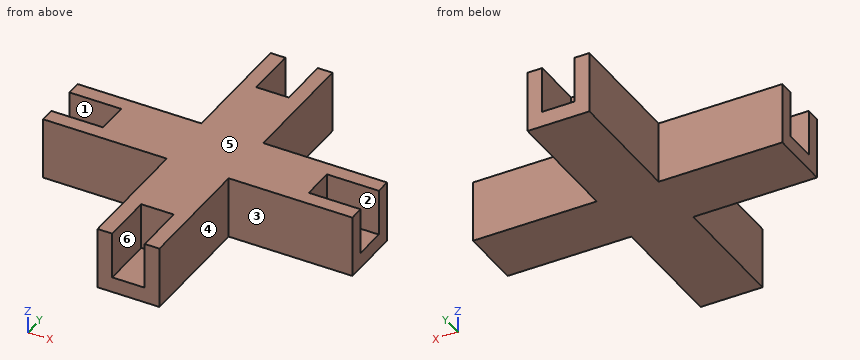
```python
from build123d import *

# Parameters (mm, degrees)
PAD322_DEPTH            = 1
PAD323_DEPTH            = 3
PAD324_DEPTH            = 3
BODY054_PLACEMENT_ANGLE = 180


with BuildPart() as part:
    # Sketch479 → Pad322 (new body)
    with BuildSketch(Plane.XY.offset(-28)):
        Polygon((-2, 2), (-2, 10), (2, 10), (2, 2), (10, 2), (10, -2), (2, -2), (2, -10), (-2, -10), (-2, -2), (-10, -2), (-10, 2), align=None)
    extrude(amount=PAD322_DEPTH)

    # Sketch480 (on Face13 of Pad322) → Pad323 (join)
    with BuildSketch(Plane(origin=(0, 0, -28), x_dir=(1, 0, 0), z_dir=(0, 0, -1))):
        Polygon((-2, 10), (-2, 2), (-10, 2), (-10, 1.05), (-1.05, 1.05), (-1.05, 10), align=None)
        Polygon((-10, -2), (-2, -2), (-2, -10), (-1.05, -10), (-1.05, -1.05), (-10, -1.05), align=None)
        Polygon((2, -10), (2, -2), (10, -2), (10, -1.05), (1.05, -1.05), (1.05, -10), align=None)
        Polygon((10, 2), (2, 2), (2, 10), (1.05, 10), (1.05, 1.05), (10, 1.05), align=None)
    extrude(amount=PAD323_DEPTH)

    # Sketch481 (on Face3 of Pad323) → Pad324 (join)
    with BuildSketch(Plane(origin=(0, 0, -28), x_dir=(1, 0, 0), z_dir=(0, 0, -1))):
        Polygon((-6.65, 1.05), (-6.65, -1.05), (-1.05, -1.05), (-1.05, -6.65), (1.05, -6.65), (1.05, -1.05), (6.65, -1.05), (6.65, 1.05), (1.05, 1.05), (1.05, 6.65), (-1.05, 6.65), (-1.05, 1.05), align=None)
    extrude(amount=PAD324_DEPTH)


with BuildPart() as part_1:
    # Body054 placement: moved
    add(part.part.moved(Location((97.37, 9.65, -44))).rotate(Axis((97.37, 9.65, -44), (1, 0, 0)), BODY054_PLACEMENT_ANGLE))


solid = part_1.part
```
Verification items for the finished model (mm, model axes). Face numbers are marked on the shaded views. A direction names the side the tool comes from. Round coordinates to 2 decimals unless told otherwise and drop trailing zeros. Write each loop counter-clockwise with the first axis right and the second up, starting at its lowest first coordinate (ties: lowest second). Pieces come first, ordered by that corner, then holes.
1. Scan lines: L1, parallel to Y at x = 104.5, z = -15.65; L2, parallel to X at y = 2, z = -14.55; L3, parallel to X at y = 18.5, z = -16.25. Record each from-to range of solid material in increasing order.
2. Section check C-C on y = 2. Enter the section's corners in (x, z), plus the area to 3 significant figures.
3. Gauge pin test, flat ends, axial feed: P1, Ø1, axis at x = 93, y = 6.5, coming from the -Z side; P2, Ø1.7, axis at x = 97.5, y = 17.5, coming from the +Z side; P3, Ø0.6, axis at y = 9.5, z = -14, coming from the -X side; P4, Ø4, axis at x = 93.5, y = 13, coming from the +Z side. Record the tip position at first contact, or that the pin passes through.
4. Section check D-D on x = 94.5. Enter the section's corners in (y, z), plus the area to 3 significant figures.
5. Section check A-A on x = 98. Enter the section's corners in (y, z).
6. Draft check along X on the marked faces 4, 5 and 6. Enter one of: +X half, -X half, draft (parallel to the pull), parting line (faces both ways), or undercut.
7. Access from +Z, -Z, +X, -X, +Y, -Y to the whole of each face (thin tool, end or side, straight path). Record for the marked faces 1, 2 and 3.
8. Section check B-B on z = -14.1. Enter the section's corners in (x, y), plus the area to 3 significant figures.
Answer:
1. L1: y = 7.65 to 8.6, 10.7 to 11.65
1. L2: x = 95.37 to 96.32, 98.42 to 99.37
1. L3: x = 95.37 to 99.37
2. outline: (95.37, -17) - (99.37, -17) - (99.37, -13) - (98.42, -13) - (98.42, -16) - (96.32, -16) - (96.32, -13) - (95.37, -13) - close
2. area: 9.70 mm2
3. P1: passes through
3. P2: stops at z = -16
3. P3: stops at x = 90.72
3. P4: stops at z = -13
4. outline: (7.65, -17) - (11.65, -17) - (11.65, -13) - (7.65, -13) - close
4. area: 16.0 mm2
5. outline: (-0.35, -17) - (19.65, -17) - (19.65, -16) - (16.3, -16) - (16.3, -13) - (3, -13) - (3, -16) - (-0.35, -16) - close
6. face 4: +X half
6. face 5: draft
6. face 6: undercut
7. face 1: +Z, -X
7. face 2: +Z, +X
7. face 3: +Z, -Z, +X, -Y
8. outline: (87.37, 7.65) - (95.37, 7.65) - (95.37, -0.35) - (96.32, -0.35) - (96.32, 3) - (98.42, 3) - (98.42, -0.35) - (99.37, -0.35) - (99.37, 7.65) - (107.37, 7.65) - (107.37, 8.6) - (104.02, 8.6) - (104.02, 10.7) - (107.37, 10.7) - (107.37, 11.65) - (99.37, 11.65) - (99.37, 19.65) - (98.42, 19.65) - (98.42, 16.3) - (96.32, 16.3) - (96.32, 19.65) - (95.37, 19.65) - (95.37, 11.65) - (87.37, 11.65) - (87.37, 10.7) - (90.72, 10.7) - (90.72, 8.6) - (87.37, 8.6) - close
8. area: 116 mm2
